Design review of the part built by this model. Coordinates are the model's own, in mm. A direction names the side the tool comes from. Round coordinates to 2 decimals unless told otherwise and drop trailing zeros. Loops run counter-clockwise (first coordinate to the right, second up) from the corner with the lowest first, then second, coordinate; pieces in that order, holes last. Notation, with made-up numbers: (83, -37) - (108, -37) arc R17 cw to (108, -25) - close; hole circle Ø9 at (68.5, 32.25). An arc over 180 degrees is marked (long way). Answer as CSV lines item,"result". Start each with the question number.
(1) Consider section A-A (z = 16.5). Give the boundary of the cut face in (x, y).
(2) For P1, Ø4, axis at x = -15, z = 40, coming from the -Y side; P2, Ø16, axis at x = -12, y = -20.5, coming from the +Z side, all flat-tipped, find the tip position at first contact; note any pin that passes through.
(3) Wall thickness on L1, parallel to X at y = -53, z = 6; L2, parallel to Z at x = 9.5, y = 23; L3, parallel to Y at x = 11.5, z = 12: over which ranges is each line inside the solid? List them lowest first.
(4) Consider section D-D (z = 27.5). Give the boundary of the cut face in (x, y).
(5) Consider section B-B (y = 31). Give the boundary of the cut face in (x, z).
(6) Consider section C-C (x = 16). Give the boundary of the cut face in (y, z), and give its area (4 significant figures).
(7) Mouldability with a two-part tool opening along Z and no side actions: class faces 4 (the flat face through (-6, -75, 18)), 5 (the flat face through (-20, -13, 10)), 6 (the flat face through (0, 1, 0)) as released by +Z, released by -Z, zero draft, split by the parting line, or undercut.
(8) For faces 1 (the flat face through (-15, -12, 25)), 2 (the flat face through (5, -13, 20)), 3 (the flat face through (0, -13, 5)), list the 3-axis set-ups (+Z, -Z, +X, -X, +Y, -Y) from which the entire face can be reached by the end or side of a thin tool; tool diameter is ignored.
from build123d import *

# Parameters (mm, degrees)
F0_W     = 50
F0_H     = 150
F1_DEPTH = 25
F3_DEPTH = 125
F5_DEPTH = 25


with BuildPart() as f1:
    # F0 (on Top) → F1 (new body)
    with BuildSketch(Plane.XY):
        Rectangle(F0_W, F0_H)
    extrude(amount=F1_DEPTH)

    # F2 (on face) → F3 (cut)
    with BuildSketch(Plane.XZ.offset(75)):
        Polygon((5, 25), (0, 25), (-5, 25), (-5, 15), (-20, 15), (-20, 5), (0, 5), (20, 5), (20, 15), (5, 15), align=None)
    extrude(amount=-F3_DEPTH, mode=Mode.SUBTRACT)

    # F4 (on face) → F5 (join)
    with BuildSketch(Plane.XY.offset(25)):
        Polygon((-25, 50), (-5, 50), (5, 50), (25, 50), (25, 75), (-25, 75), align=None)
    extrude(amount=F5_DEPTH)


solid = f1.part
Determined:
1,outline,"(-25, -75) - (-5, -75) - (-5, 50) - (5, 50) - (5, -75) - (25, -75) - (25, 75) - (-25, 75) - close"
2,P1,"stops at y = 50"
2,P2,"stops at z = 25"
3,L1,"x = -25 to -20, 20 to 25"
3,L2,"z = 0 to 5, 15 to 25"
3,L3,"y = 50 to 75"
4,outline,"(-25, 50) - (25, 50) - (25, 75) - (-25, 75) - close"
5,outline,"(-25, 0) - (25, 0) - (25, 25) - (5, 25) - (5, 15) - (20, 15) - (20, 5) - (-20, 5) - (-20, 15) - (-5, 15) - (-5, 25) - (-25, 25) - close"
6,outline,"(-75, 0) - (75, 0) - (75, 50) - (50, 50) - (50, 25) - (-75, 25) - (-75, 15) - (50, 15) - (50, 5) - (-75, 5) - close"
6,area,"3,125 mm^2"
7,face 4,"zero draft"
7,face 5,"undercut"
7,face 6,"released by -Z"
8,face 1,"+Z, +X, -X, -Y"
8,face 2,"+Z, -Y"
8,face 3,"-Y"
